Model file for the job. Use its own axes, mm. A direction names the side the tool comes from. Round coordinates to 2 decimals unless told otherwise and drop trailing zeros. Order: outer loops, then holes, each group sorted by start corner. A loop starts at its lowest first (then second) coordinate and runs counter-clockwise, first axis right, second up. Notation, with made-up numbers: (64, 54) - (92, 54) arc R18 cw to (92, 72) - close; hole circle Ø6 at (-23, -29.5). An arc over 180 degrees is marked (long way). Put each result on its own line as item: value. Start each with the question number.
Item 1: Which spindle directions (+Z, -Z, +X, -X, +Y, -Y) get a long thin tool onto all of the face, cutting with end or side? Do faces 4 (the face through (-63, -55, 5)), 5 (the face through (-48, -75, 5)), 6 (the face through (-48, -65, 9)). Say none if no direction does.
Item 2: Saw through at A-A on x = -41.25. List the corners of the cut face in (y, z).
Item 3: Pin check, flat tips, straight feed: pin 1 Ø6.5 at (x, y) = (-34.5, -65) entering from +Z; pin 2 Ø4.5 at (x, z) = (-62.5, 5) entering from +Y; pin 3 Ø0.8 at (x, z) = (-53.5, 9.5) entering from +Y. Stop position of each tip, or through.
Item 4: Mould opens along Y. For faces 1 (the face through (-18.247, 0.143, 4.93)), 2 (the face through (-69.4, -56.43, 4.93)), 3 (the face through (42, -91.75, 5)) say: pulls with the +Y half, pulls with the -Y half, needs draft (parallel to the pull), parting line crosses it, or undercut.
Item 5: Probe probe 1 along Y at (x, z) = (-34.5, 6.25); probe 2 along X at (y, z) = (-2, 1); probe 3 along X at (y, z) = (-16.5, 8.25). List the from-to ranges inside material, lowest first.
Item 6: Saw through at B-B on z = 7. State how many separate pieces and enclosed holes the cut face has, plus the area to 3 significant figures.
Item 7: Saw through at D-D on y = -65. List the corners of the cut face in (x, z).
Item 8: Saw through at C-C on y = 0. List the corners of the cut face in (x, z).
```python
from build123d import *

# Parameters (mm, degrees)
F0_R     = 2.1
F0_R_2   = 5.5
F0_R_3   = 2.4
F0_R_4   = 3.75
F0_R_5   = 3.25
F1_DEPTH = 10
F2_W     = 39.5
F2_H     = 12.6
F2_R     = 2.074687
F2_R_2   = 2.038572
F3_DEPTH = 1


with BuildPart() as f1:
    # F0 (on Top) → F1 (new body)
    with BuildSketch(Plane.XY):
        with BuildLine():
            ThreePointArc((55, 86.75), (53.535534, 90.285534), (50, 91.75))
            Line((50, 91.75), (-50, 91.75))
            ThreePointArc((-50, 91.75), (-53.535534, 90.285534), (-55, 86.75))
            Line((-55, 86.75), (-55, -50))
            ThreePointArc((-55, -50), (-56.464466, -53.535534), (-60, -55))
            Line((-60, -55), (-65.9, -55))
            ThreePointArc((-65.9, -55), (-69.435534, -56.464466), (-70.9, -60))
            Line((-70.9, -60), (-70.9, -70))
            ThreePointArc((-70.9, -70), (-69.435534, -73.535534), (-65.9, -75))
            Line((-65.9, -75), (-60, -75))
            Line((-60, -75), (-30, -75))
            ThreePointArc((-30, -75), (-26.464466, -76.464466), (-25, -80))
            Line((-25, -80), (-25, -86.75))
            ThreePointArc((-25, -86.75), (-23.535534, -90.285534), (-20, -91.75))
            Line((-20, -91.75), (-8.616731, -91.75))
            ThreePointArc((-8.616731, -91.75), (15, -43.25), (38.616731, -91.75))
            Line((38.616731, -91.75), (45, -91.75))
            ThreePointArc((45, -91.75), (52.071068, -88.821068), (55, -81.75))
            Line((55, -81.75), (55, -68.25))
            Line((55, -68.25), (55, 86.75))
        make_face()
        with Locations((-60.9, -65)):
            Circle(F0_R, mode=Mode.SUBTRACT)
        with Locations((-34.5, -65)):
            Circle(F0_R, mode=Mode.SUBTRACT)
        with Locations((-25, -10)):
            Circle(F0_R_2, mode=Mode.SUBTRACT)
        with Locations((-10, -15)):
            Circle(F0_R_3, mode=Mode.SUBTRACT)
        with Locations((40, -15)):
            Circle(F0_R_3, mode=Mode.SUBTRACT)
        with Locations((49, -10)):
            Circle(F0_R_2, mode=Mode.SUBTRACT)
        with Locations((-41.25, 35)):
            Circle(F0_R_4, mode=Mode.SUBTRACT)
        with Locations((-15, 0)):
            Circle(F0_R_5, mode=Mode.SUBTRACT)
        with Locations((-41.25, 78)):
            Circle(F0_R_4, mode=Mode.SUBTRACT)
        with Locations((45, 0)):
            Circle(F0_R_5, mode=Mode.SUBTRACT)
        with Locations((41.25, 35)):
            Circle(F0_R_4, mode=Mode.SUBTRACT)
        with Locations((41.25, 78)):
            Circle(F0_R_4, mode=Mode.SUBTRACT)
    extrude(amount=F1_DEPTH)

    # F2 (on face) → F3 (cut)
    with BuildSketch(Plane.XY.offset(10)):
        with Locations((-47.7, -65)):
            Rectangle(F2_W, F2_H)
        with Locations((-60.9, -65)):
            Circle(F2_R, mode=Mode.SUBTRACT)
        with Locations((-34.5, -65)):
            Circle(F2_R_2, mode=Mode.SUBTRACT)
    extrude(amount=-F3_DEPTH, mode=Mode.SUBTRACT)


solid = f1.part
```
Results found:
1. face 4: +Z, -Z, -X, +Y
1. face 5: +Z, -Z, -X, -Y
1. face 6: +Z
2. outline: (-75, 0) - (31.25, 0) - (31.25, 10) - (-58.7, 10) - (-58.7, 9) - (-71.3, 9) - (-71.3, 10) - (-75, 10) - close; (38.75, 0) - (74.25, 0) - (74.25, 10) - (38.75, 10) - close; (81.75, 0) - (91.75, 0) - (91.75, 10) - (81.75, 10) - close
3. pin 1: stops at z = 9
3. pin 2: stops at y = -55
3. pin 3: stops at y = 90.67
4. face 1: undercut
4. face 2: pulls with the +Y half
4. face 3: pulls with the -Y half
5. probe 1: y = -75 to -67.1, -62.9 to 91.75
5. probe 2: x = -55 to -17.56, -12.44 to 42.44, 47.56 to 55
5. probe 3: x = -55 to -11.87, -8.13 to 38.13, 41.87 to 55
6. separate pieces: 1
6. enclosed holes: 12
6. area: 17,000 mm²
7. outline: (-70.9, 0) - (-63, 0) - (-63, 9) - (-67.45, 9) - (-67.45, 10) - (-70.9, 10) - close; (-58.8, 0) - (-36.6, 0) - (-36.6, 9) - (-58.8, 9) - close; (-32.4, 0) - (-13.84, 0) - (-13.84, 10) - (-27.95, 10) - (-27.95, 9) - (-32.4, 9) - close; (43.84, 0) - (55, 0) - (55, 10) - (43.84, 10) - close
8. outline: (-55, 0) - (-18.25, 0) - (-18.25, 10) - (-55, 10) - close; (-11.75, 0) - (41.75, 0) - (41.75, 10) - (-11.75, 10) - close; (48.25, 0) - (55, 0) - (55, 10) - (48.25, 10) - close
